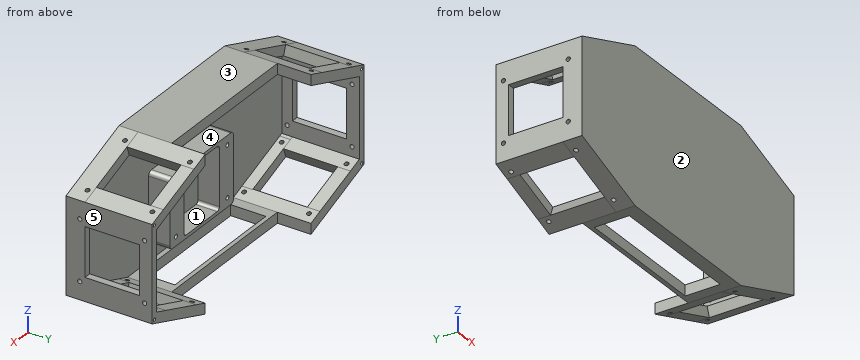
```python
from build123d import *

# Parameters (mm, degrees)
BOSS_EXTRUDE1_DEPTH     = 8
SKETCH2_W               = 10.5
SKETCH2_H               = 10
BOSS_EXTRUDE2_DEPTH     = 37.5
SKETCH4_W               = 128.649180674
SKETCH4_H               = 10
BOSS_EXTRUDE4_DEPTH     = 4.5
BOSS_EXTRUDE5_DEPTH     = 10
SKETCH6_W               = 149.649180674
SKETCH6_H               = 10
BOSS_EXTRUDE6_DEPTH     = 4
SKETCH7_R               = 2
CUT_EXTRUDE1_DEPTH      = 9.396926
MIRROR2_COPY_1_SKETCH_R = 2
MIRROR2_COPY_1_DEPTH    = 9.396926
SKETCH8_R               = 2
CUT_EXTRUDE2_DEPTH      = 75.17541
BOSS_EXTRUDE8_DEPTH     = 63
SKETCH10_R              = 2
CUT_EXTRUDE3_DEPTH      = 9.396926
MIRROR5_COPY_1_SKETCH_R = 2
MIRROR5_COPY_1_DEPTH    = 9.396926
SKETCH11_R              = 2
CUT_EXTRUDE4_DEPTH      = 75.17541
SKETCH12_W              = 6.577848346
SKETCH12_H              = 46
BOSS_EXTRUDE9_DEPTH     = 12
BOSS_EXTRUDE10_DEPTH    = 20
SKETCH14_R              = 2
CUT_EXTRUDE5_DEPTH      = 10
SKETCH15_W              = 149.649180674
SKETCH15_H              = 10
BOSS_EXTRUDE11_DEPTH    = 41.5
SKETCH17_R              = 1.5
CUT_EXTRUDE6_DEPTH      = 10


with BuildPart() as part:
    # Sketch1 → Boss-Extrude1 (new body)
    with BuildSketch(Plane(origin=(0, 0, 0), x_dir=(1, 0, 0), z_dir=(0, 1, 0))):
        Polygon((-150, 45), (-150, -45), (-74.824590337, -72.361611466), (74.824590337, -72.361611466), (150, -45), (150, 45), (74.824590337, 72.361611466), (-74.824590337, 72.361611466), align=None)
    extrude(amount=BOSS_EXTRUDE1_DEPTH)

    # Sketch2 → Boss-Extrude2 (add)
    with BuildSketch(Plane(origin=(0, 8, 0), x_dir=(1, 0, 0), z_dir=(0, 1, 0))):
        with Locations((69.574590337, 67.361611466)):
            Rectangle(SKETCH2_W, SKETCH2_H)
        with Locations((-69.574590337, 67.361611466)):
            Rectangle(SKETCH2_W, SKETCH2_H)
    extrude(amount=BOSS_EXTRUDE2_DEPTH)

    # Sketch4 → Boss-Extrude4 (add)
    with BuildSketch(Plane(origin=(0, 8, 0), x_dir=(1, 0, 0), z_dir=(0, 1, 0))):
        with Locations((0, 67.361611466)):
            Rectangle(SKETCH4_W, SKETCH4_H)
    extrude(amount=BOSS_EXTRUDE4_DEPTH)

    # Sketch5 → Boss-Extrude5 (add)
    with BuildSketch(Plane(origin=(0, 8, 0), x_dir=(1, 0, 0), z_dir=(0, 1, 0))):
        Polygon((-74.824590337, 62.361611466), (-87.040594407, 57.915349603), (-140.603073792, 38.420201433), (-143.422151654, 37.394141003), (-143.422151654, -37.394141003), (-140.603073792, -38.420201433), (-87.040594407, -57.915349603), (-74.824590337, -62.361611466), (-74.824590337, -72.361611466), (-150, -45), (-150, 45), (-74.824590337, 72.361611466), align=None)
        Polygon((150, 45), (150, -45), (74.824590337, -72.361611466), (74.824590337, -62.361611466), (87.040594407, -57.915349603), (140.603073792, -38.420201433), (143.422151654, -37.394141003), (143.422151654, 37.394141003), (140.603073792, 38.420201433), (87.040594407, 57.915349603), (74.824590337, 62.361611466), (74.824590337, 72.361611466), align=None)
    extrude(amount=BOSS_EXTRUDE5_DEPTH)

    # Sketch6 → Boss-Extrude6 (add)
    with BuildSketch(Plane(origin=(0, 45.5, 0), x_dir=(1, 0, 0), z_dir=(0, 1, 0))):
        with Locations((0, 67.361611466)):
            Rectangle(SKETCH6_W, SKETCH6_H)
    extrude(amount=BOSS_EXTRUDE6_DEPTH)

    # Sketch7 → Cut-Extrude1 (cut)
    with BuildSketch(Plane(origin=(32.009387984, 0, -87.945070697), x_dir=(-0.939692621, 0, -0.342020143), z_dir=(0.342020143, 0, -0.939692621))):
        with Locations((-113.852986668, 13)):
            Circle(SKETCH7_R)
        with Locations((-57.272986668, 13)):
            Circle(SKETCH7_R)
    cut_extrude1 = extrude(amount=-CUT_EXTRUDE1_DEPTH, mode=Mode.SUBTRACT)

    # Mirror1: Cut-Extrude1 across plane
    add(cut_extrude1.mirror(Plane(origin=(0, 0, 0), x_dir=(0, 0, 1), z_dir=(1, 0, 0))), mode=Mode.SUBTRACT)

    # Mirror2: Cut-Extrude1 across plane
    add(cut_extrude1.mirror(Plane(origin=(0, 0, 0), x_dir=(1, 0, 0), z_dir=(0, 0, -1))), mode=Mode.SUBTRACT)

    # Mirror2 copy 1 sketch → Mirror2 copy 1 (cut)
    with BuildSketch(Plane(origin=(-32.009387984, 0, 87.945070697), x_dir=(0.939692621, 0, 0.342020143), z_dir=(-0.342020143, 0, 0.939692621))):
        with Locations((-113.852986668, 13)):
            Circle(MIRROR2_COPY_1_SKETCH_R)
        with Locations((-57.272986668, 13)):
            Circle(MIRROR2_COPY_1_SKETCH_R)
    extrude(amount=-MIRROR2_COPY_1_DEPTH, mode=Mode.SUBTRACT)

    # Sketch8 → Cut-Extrude2 (cut)
    with BuildSketch(Plane(origin=(150, 0, 0), x_dir=(0, 0, -1), z_dir=(1, 0, 0))):
        with Locations((-28.29, 13)):
            Circle(SKETCH8_R)
        with Locations((28.29, 13)):
            Circle(SKETCH8_R)
    cut_extrude2 = extrude(amount=-CUT_EXTRUDE2_DEPTH, mode=Mode.SUBTRACT)

    # Mirror3: Cut-Extrude2 across plane
    add(cut_extrude2.mirror(Plane(origin=(0, 0, 0), x_dir=(0, 0, 1), z_dir=(1, 0, 0))), mode=Mode.SUBTRACT)

    # Sketch9 → Boss-Extrude8 (add)
    with BuildSketch(Plane(origin=(0, 18, 0), x_dir=(1, 0, 0), z_dir=(0, 1, 0))):
        Polygon((143.422151654, 23), (150, 23), (150, 45), (134.025225447, 50.814342437), (130.811287398, 41.984120221), (143.422151654, 37.394141003), align=None)
        Polygon((74.824590337, 72.361611466), (90.79936489, 66.54726903), (87.585426842, 57.717046814), (74.824590337, 62.361611466), align=None)
        Polygon((-74.824590337, 62.361611466), (-74.824590337, 72.361611466), (-90.79936489, 66.54726903), (-87.585426842, 57.717046814), align=None)
        Polygon((-143.422151654, 37.394141003), (-143.422151654, 23), (-150, 23), (-150, 45), (-134.025225447, 50.814342437), (-130.811287398, 41.984120221), align=None)
        Polygon((143.422151654, -37.394141003), (143.422151654, -23), (150, -23), (150, -45), (134.025225447, -50.814342437), (130.811287398, -41.984120221), align=None)
        Polygon((-143.422151654, -23), (-150, -23), (-150, -45), (-134.025225447, -50.814342437), (-130.811287398, -41.984120221), (-143.422151654, -37.394141003), align=None)
        Polygon((-74.824590337, -72.361611466), (-90.79936489, -66.54726903), (-87.585426842, -57.717046814), (-74.824590337, -62.361611466), align=None)
        Polygon((74.824590337, -62.361611466), (74.824590337, -72.361611466), (90.79936489, -66.54726903), (87.585426842, -57.717046814), align=None)
    extrude(amount=BOSS_EXTRUDE8_DEPTH)

    # Sketch10 → Cut-Extrude3 (cut)
    with BuildSketch(Plane(origin=(32.009387984, 0, -87.945070697), x_dir=(-0.939692621, 0, -0.342020143), z_dir=(0.342020143, 0, -0.939692621))):
        with Locations((-113.852986668, 74)):
            Circle(SKETCH10_R)
        with Locations((-57.272986668, 74)):
            Circle(SKETCH10_R)
    cut_extrude3 = extrude(amount=-CUT_EXTRUDE3_DEPTH, mode=Mode.SUBTRACT)

    # Mirror4: Cut-Extrude3 across plane
    add(cut_extrude3.mirror(Plane(origin=(0, 0, 0), x_dir=(0, 0, 1), z_dir=(1, 0, 0))), mode=Mode.SUBTRACT)

    # Mirror5: Cut-Extrude3 across plane
    add(cut_extrude3.mirror(Plane(origin=(0, 0, 0), x_dir=(1, 0, 0), z_dir=(0, 0, -1))), mode=Mode.SUBTRACT)

    # Mirror5 copy 1 sketch → Mirror5 copy 1 (cut)
    with BuildSketch(Plane(origin=(-32.009387984, 0, 87.945070697), x_dir=(0.939692621, 0, 0.342020143), z_dir=(-0.342020143, 0, 0.939692621))):
        with Locations((-113.852986668, 74)):
            Circle(MIRROR5_COPY_1_SKETCH_R)
        with Locations((-57.272986668, 74)):
            Circle(MIRROR5_COPY_1_SKETCH_R)
    extrude(amount=-MIRROR5_COPY_1_DEPTH, mode=Mode.SUBTRACT)

    # Sketch11 → Cut-Extrude4 (cut)
    with BuildSketch(Plane(origin=(150, 0, 0), x_dir=(0, 0, -1), z_dir=(1, 0, 0))):
        with Locations((-28.29, 74)):
            Circle(SKETCH11_R)
        with Locations((28.29, 74)):
            Circle(SKETCH11_R)
    cut_extrude4 = extrude(amount=-CUT_EXTRUDE4_DEPTH, mode=Mode.SUBTRACT)

    # Mirror6: Cut-Extrude4 across plane
    add(cut_extrude4.mirror(Plane(origin=(0, 0, 0), x_dir=(0, 0, 1), z_dir=(1, 0, 0))), mode=Mode.SUBTRACT)

    # Sketch12 → Boss-Extrude9 (add)
    with BuildSketch(Plane(origin=(0, 81, 0), x_dir=(1, 0, 0), z_dir=(0, 1, 0))):
        Polygon((130.811287398, 41.984120221), (87.585426842, 57.717046814), (90.79936489, 66.54726903), (134.025225447, 50.814342437), align=None)
        with Locations((146.711075827, 0)):
            Rectangle(SKETCH12_W, SKETCH12_H)
        Polygon((134.025225447, -50.814342437), (130.811287398, -41.984120221), (87.585426842, -57.717046814), (90.79936489, -66.54726903), align=None)
        Polygon((-130.811287398, -41.984120221), (-87.585426842, -57.717046814), (-90.79936489, -66.54726903), (-134.025225447, -50.814342437), align=None)
        with Locations((-146.711075827, 0)):
            Rectangle(SKETCH12_W, SKETCH12_H)
        Polygon((-134.025225447, 50.814342437), (-130.811287398, 41.984120221), (-87.585426842, 57.717046814), (-90.79936489, 66.54726903), align=None)
    extrude(amount=-BOSS_EXTRUDE9_DEPTH)

    # Sketch13 → Boss-Extrude10 (add)
    with BuildSketch(Plane(origin=(0, 8, 0), x_dir=(1, 0, 0), z_dir=(0, 1, 0))):
        with BuildLine():
            Line((-41, 46.231611466), (-29, 46.231611466))
            Line((-29, 46.231611466), (29, 46.231611466))
            Line((29, 46.231611466), (41, 46.231611466))
            ThreePointArc((41, 46.231611466), (43.828427125, 45.060038591), (45, 42.231611466))
            Line((45, 42.231611466), (45, -14.768388534))
            ThreePointArc((45, -14.768388534), (43.828427125, -17.596815659), (41, -18.768388534))
            Line((41, -18.768388534), (29, -18.768388534))
            Line((29, -18.768388534), (-29, -18.768388534))
            Line((-29, -18.768388534), (-41, -18.768388534))
            ThreePointArc((-41, -18.768388534), (-43.828427125, -17.596815659), (-45, -14.768388534))
            Line((-45, -14.768388534), (-45, 42.231611466))
            ThreePointArc((-45, 42.231611466), (-43.828427125, 45.060038591), (-41, 46.231611466))
        make_face()
        with BuildLine():
            Line((-25, 40.231611466), (-25, -12.768388534))
            ThreePointArc((-25, -12.768388534), (-24.121320344, -14.889708878), (-22, -15.768388534))
            Line((-22, -15.768388534), (22, -15.768388534))
            ThreePointArc((22, -15.768388534), (24.121320344, -14.889708878), (25, -12.768388534))
            Line((25, -12.768388534), (25, 40.231611466))
            ThreePointArc((25, 40.231611466), (24.121320344, 42.35293181), (22, 43.231611466))
            Line((22, 43.231611466), (-22, 43.231611466))
            ThreePointArc((-22, 43.231611466), (-24.121320344, 42.35293181), (-25, 40.231611466))
        make_face(mode=Mode.SUBTRACT)
    extrude(amount=BOSS_EXTRUDE10_DEPTH)

    # Sketch14 → Cut-Extrude5 (cut)
    with BuildSketch(Plane(origin=(0, 28, 0), x_dir=(1, 0, 0), z_dir=(0, 1, 0))):
        with Locations((-36.37, 37.606611466)):
            Circle(SKETCH14_R)
        with Locations((-36.37, -10.143388534)):
            Circle(SKETCH14_R)
    cut_extrude5 = extrude(amount=-CUT_EXTRUDE5_DEPTH, mode=Mode.SUBTRACT)

    # Mirror7: Cut-Extrude5 across plane
    add(cut_extrude5.mirror(Plane(origin=(0, 0, 0), x_dir=(0, 0, 1), z_dir=(1, 0, 0))), mode=Mode.SUBTRACT)

    # Sketch15 → Boss-Extrude11 (add)
    with BuildSketch(Plane(origin=(0, 8, 0), x_dir=(1, 0, 0), z_dir=(0, 1, 0))):
        with Locations((0, -67.361611466)):
            Rectangle(SKETCH15_W, SKETCH15_H)
    extrude(amount=BOSS_EXTRUDE11_DEPTH)

    # Sketch17 → Cut-Extrude6 (cut)
    with BuildSketch(Plane(origin=(0, 81, 0), x_dir=(1, 0, 0), z_dir=(0, 1, 0))):
        with Locations((146.723391823, -42.705694255)):
            Circle(SKETCH17_R)
        with Locations((146.723391823, 42.705694255)):
            Circle(SKETCH17_R)
        with Locations((-146.723391823, 42.705694255)):
            Circle(SKETCH17_R)
        with Locations((-146.723391823, -42.705694255)):
            Circle(SKETCH17_R)
    extrude(amount=-CUT_EXTRUDE6_DEPTH, mode=Mode.SUBTRACT)


solid = part.part
```
Model file for the job. Use its own axes, mm. Face numbers are marked on the shaded views. A direction names the side the tool comes from. Coordinates: 2 decimals unless noted, no trailing zeros. Loops run counter-clockwise (first coordinate to the right, second up) from the corner with the lowest first, then second, coordinate; pieces in that order, holes last. Notation, with made-up numbers: (71.25, 32) - (95.25, 32) arc R17 cw to (95.25, 39) - close; hole circle Ø2 at (51, 25). An arc over 180 degrees is marked (long way). Write item = value, one per line. Start each with the question number.
Item 1: Wall check: probe 1 along Z at (x, y) = (36, 23); probe 2 along Y at (x, z) = (-121, 47); probe 3 along Y at (x, z) = (-148.5, -28.29). Give the ranges that are in metal, low to high. Write a range as [from, to].
Item 2: Drop flat-ended pins along their axis: pin 1 Ø1 at (x, y) = (20, 32) entering from -Z; pin 2 Ø6 at (x, z) = (-110, 10) entering from -Y; pin 3 Ø3 at (y, z) = (57.5, 68) entering from -X; pin 4 Ø2 at (x, z) = (88, -42) entering from +Y. Give the stop position or say it passes through.
Item 3: Pull direction X, two halves, no side cores. Call the marked faces 3, 4 and 5: +X half, -X half, draft (parallel to the pull), parting line (faces both ways), or undercut.
Item 4: Saw through at A-A, the plane z = 4.5. List the corners of the cut face in (x, y).
Item 5: 3-axis set-ups, long thin cutter, end or side, ignore diameter. For the marked faces 1 and 2: which of +Z, -Z, +X, -X, +Y, -Y reach the whole face in a straight line?
Answers:
q1.probe_1 = [-46.23, -39.57], [-35.64, 8.18], [12.11, 18.77], [62.36, 72.36]
q1.probe_2 = [0, 18], [69, 81]
q1.probe_3 = [0, 11], [15, 72], [76, 81]
q2.pin_1 = 62.36
q2.pin_2 = 0
q2.pin_3 = -90.8
q2.pin_4 = 8
q3.face_3 = draft
q3.face_4 = undercut
q3.face_5 = +X half
q4.outline = (-150, 0) - (150, 0) - (150, 18) - (143.42, 18) - (143.42, 8) - (45, 8) - (45, 28) - (25, 28) - (25, 8) - (-25, 8) - (-25, 28) - (-45, 28) - (-45, 8) - (-143.42, 8) - (-143.42, 18) - (-150, 18) - close; (-150, 69) - (-143.42, 69) - (-143.42, 81) - (-150, 81) - close; (143.42, 69) - (150, 69) - (150, 81) - (143.42, 81) - close
q5.face_1 = +Y
q5.face_2 = +Z, -Z, +X, -X, -Y
